The listing builds one solid part. Answer for the finished solid, in the listing's coordinates (mm). Round coordinates to 2 decimals unless told otherwise and drop trailing zeros. Loops run counter-clockwise (first coordinate to the right, second up) from the corner with the lowest first, then second, coordinate; pieces in that order, holes last. Notation, with made-up numbers: (-14, 51.25) - (-5, 51.25) arc R31 cw to (-5, 86.25) - close; hole circle Ø9 at (23, 79). An arc over 180 degrees is marked (long way). One line per question, with ' | ' between items. Start each with the question number.
from build123d import *

# Parameters (mm, degrees)
F1_DEPTH = 6.1
F3_D     = 4
F4_SIZE  = 1


with BuildPart() as f1:
    # F0 (on Top) → F1 (new body)
    with BuildSketch(Plane.XY):
        with BuildLine():
            Line((9.1, 9.1), (39.977369, 9.1))
            ThreePointArc((39.977369, 9.1), (28.991378, 28.991378), (9.1, 39.977369))
            Line((9.1, 39.977369), (9.1, 9.1))
        make_face()
    extrude(amount=F1_DEPTH)

    # F3 (through all)
    with Locations(Plane.XY.offset(6.1)):
        with Locations((14, 14), (24, 24)):
            Hole(F3_D / 2)

    # F4
    f4_edges = [f1.edges().sort_by_distance(p)[0] for p in [
        (9.1, 9.1, 3.05),
    ]]
    chamfer(f4_edges, length=F4_SIZE)


solid = f1.part
(1) Each of these flat-tipped pins is pushed along its axis until it touches: P1, Ø2, axis at y = 32.5, z = 4.5, coming from the +X side; P2, Ø1.5, axis at y = 20.5, z = 1.5, coming from the +X side; P3, Ø3, axis at y = 16, z = 5, coming from the +X side. Where does it stop, or does it pass through?
(2) Find section D-D on y = 29.5. Write down the section's boundary in (x, z), plus the area to 3 significant figures.
(3) Find section C-C on z = 4.75. Write down the section's boundary in (x, y).
(4) Find section A-A on x = 12.5. Write down the section's boundary in (y, z).
(5) Determine the mould class of faces 1 (the flat face through (25, 9.1, 3)), 2 (the cylindrical face through (29.22, 28.76, 3.01)), 3 (the cylindrical face through (14, 16, 3)) for opening direction X: pulls with the +X half, pulls with the -X half, needs draft (parallel to the pull), parting line crosses it, or undercut.
(6) Consider L1, parallel to Y at x = 14, z = 2.75; L2, parallel to Y at x = 22.5, z = 1.5; L3, parallel to X at y = 37.5, z = 1.75. Determine where each line is inside the solid, lowest interval first.
(7) Find section B-B on y = 14. Write down the section's boundary in (x, z).
Answer below:
1) P1: x = 26.24 | P2: x = 35.93 | P3: x = 38.35
2) outline: (9.1, 0) - (28.47, 0) - (28.47, 6.1) - (9.1, 6.1) - close | area: 118 mm2
3) outline: (9.1, 10.1) - (10.1, 9.1) - (39.98, 9.1) arc R41 ccw to (9.1, 39.98) - close; hole circle Ø4 at (14, 14); hole circle Ø4 at (24, 24)
4) outline: (9.1, 0) - (12.68, 0) - (12.68, 6.1) - (9.1, 6.1) - close; (15.32, 0) - (39.05, 0) - (39.05, 6.1) - (15.32, 6.1) - close
5) face 1: needs draft | face 2: pulls with the +X half | face 3: undercut
6) L1: 9.1 to 12, 16 to 38.54 | L2: 9.1 to 22.68, 25.32 to 34.27 | L3: 9.1 to 16.58
7) outline: (9.1, 0) - (12, 0) - (12, 6.1) - (9.1, 6.1) - close; (16, 0) - (38.54, 0) - (38.54, 6.1) - (16, 6.1) - close
